Check sheet for the drawn part. Datum: minimum x, y, z corner. Units: mm. A direction names the side the tool comes from. Coordinates: 2 decimals unless noted, no trailing zeros. Order: outer loops, then holes, each group sorted by start corner. A loop starts at its lowest first (then second) coordinate and runs counter-clockwise, first axis right, second up. Notation, with made-up numbers: M -33,48.25 L -21,48.25 A28 ccw -21,70.25 Z; hole C -3.75,85 d11. An arc over 180 degrees is marked long. Answer in a Markdown table with one row per item. Add a question column.
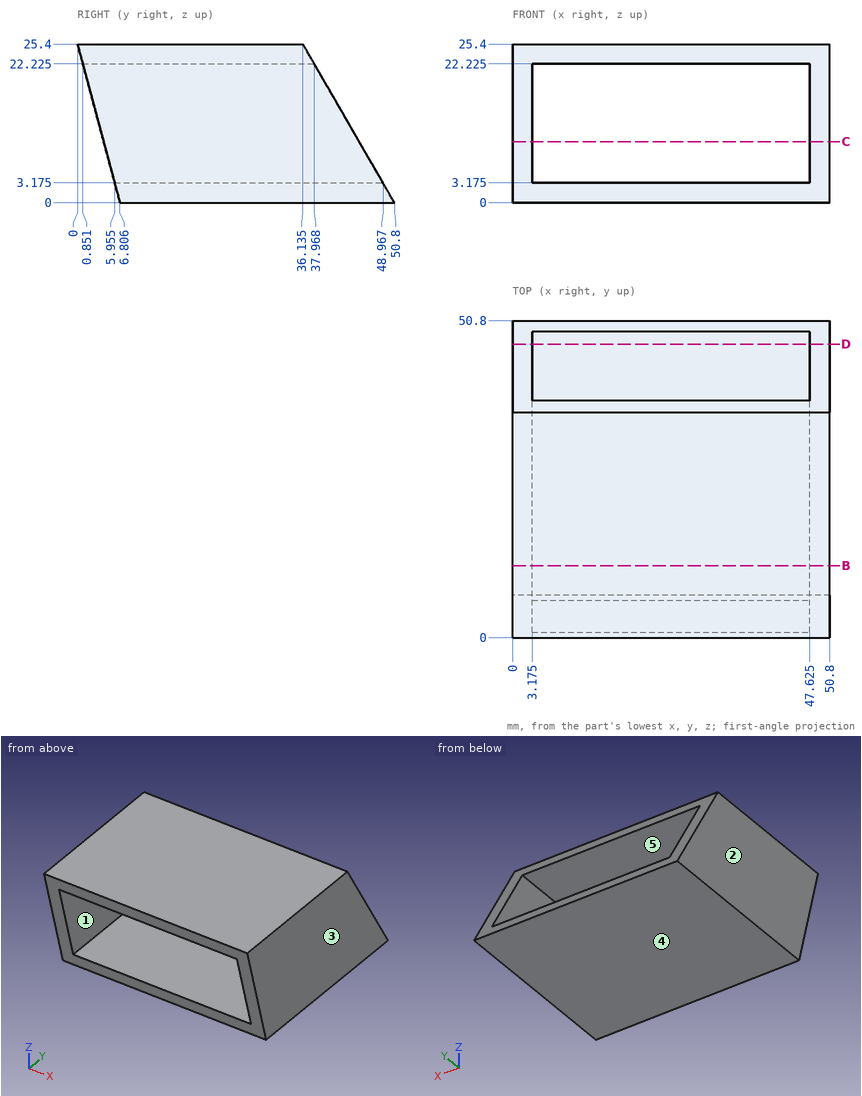
1. Section check D-D on y = 47. Enter the section's corners in (x, z) (1 decimal), then the cut area to 3 significant figures.
2. Go/stop test with flat-tipped pins: pin 1 Ø15 at (y, z) = (14.5, 11.5) entering from -X; pin 2 Ø5 at (x, z) = (39, 21) entering from -Y; pin 3 Ø5 at (x, z) = (18.5, 22.5) entering from -Y; pin 4 Ø1.5 at (x, z) = (7.5, 22.5) entering from -Y. Record where each tip stops, or that it passes through.
3. Section check B-B on y = 11.5. Enter the section's corners in (x, z) (1 decimal).
4. Release check for a two-part mould opening along X. For the marked faces 3, 4 and 5 record: released by +X, released by -X, zero draft, split by the parting line, or undercut.
5. Set-up check for the marked faces 1 and 2: record each of +Z, -Z, +X, -X, +Y, -Y from which the full face is reachable in a straight line by a thin tool's end or side.
6. Section check C-C on z = 9.75. Enter the section's corners in (x, y) (1 decimal), then the cut area to 3 significant figures.
7. Scan lines: line 1 (X direction, y = 37, z = 17.5) (1 decimal); line 2 (Z direction, x = 27.5, y = 41) (1 decimal); line 3 (Z direction, x = 12, y = 13) (1 decimal). Record each from-to range of solid material in increasing order.
Result sheet:
| question | item | result |
|---|---|---|
| 1 | outline | M 0,0 L 50.8,0 L 50.8,6.6 L 47.6,6.6 L 47.6,3.2 L 3.2,3.2 L 3.2,6.6 L 0,6.6 Z |
| 1 | area | 183 mm^2 |
| 2 | pin 1 | x = 0 |
| 2 | pin 2 | y = 0.51 |
| 2 | pin 3 | y = 0.11 |
| 2 | pin 4 | y = 0.58 |
| 3 | outline | M 0,0 L 50.8,0 L 50.8,25.4 L 0,25.4 Z; hole M 3.2,3.2 L 47.6,3.2 L 47.6,22.2 L 3.2,22.2 Z |
| 4 | face 3 | released by +X |
| 4 | face 4 | zero draft |
| 4 | face 5 | undercut |
| 5 | face 1 | +Y, -Y |
| 5 | face 2 | +Z, -Z, -X, +Y, -Y |
| 6 | outline | M 0,4.2 L 3.2,4.2 L 3.2,45.2 L 0,45.2 Z; M 47.6,4.2 L 50.8,4.2 L 50.8,45.2 L 47.6,45.2 Z |
| 6 | area | 260 mm^2 |
| 7 | line 1 | 0 to 3.2, 47.6 to 50.8 |
| 7 | line 2 | 0 to 3.2 |
| 7 | line 3 | 0 to 3.2, 22.2 to 25.4 |
